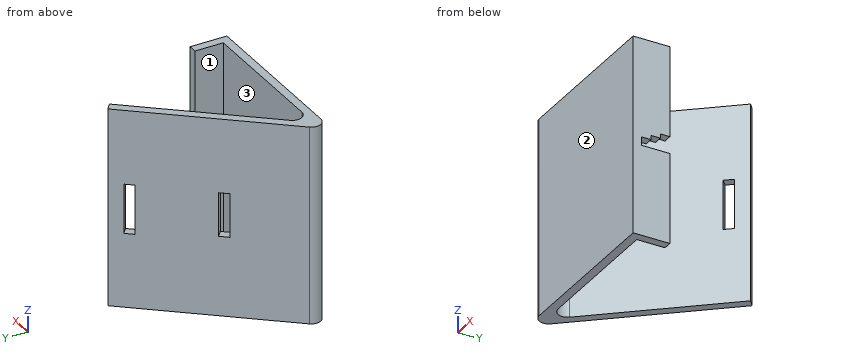
```python
from build123d import *

# Parameters (mm, degrees)
PAD_DEPTH       = 70
SKETCH001_W     = 3.5
SKETCH001_H     = 17.5
SKETCH001_H_2   = 15.5
POCKET_DEPTH    = 34.50505
POCKET001_DEPTH = 5


with BuildPart() as part:
    # Sketch → Pad (new body)
    with BuildSketch(Plane.XY):
        with BuildLine():
            Line((7.250462, 0), (65, 0))
            Line((65, 0), (65, 3))
            Line((65, 3), (65, 13))
            Line((65, 13), (62, 13))
            Line((62, 13), (62, 3))
            Line((62, 3), (13.683983, 3))
            ThreePointArc((11.094028, 8.554176), (10.619805, 4.952097), (13.683983, 3))
            Line((11.094028, 8.554176), (47.293266, 51.694748))
            Line((47.293266, 51.694748), (44.995133, 53.623111))
            Line((4.660507, 5.554176), (44.995133, 53.623111))
            ThreePointArc((4.660507, 5.554176), (4.186285, 1.952097), (7.250462, 0))
        make_face()
    extrude(amount=PAD_DEPTH)

    # Sketch001 (on Face9 of Pad) → Pocket (cut, through all)
    with BuildSketch(Plane(origin=(2.298133, -1.928363, 0), x_dir=(0.642788, 0.766044, 0), z_dir=(0.766044, -0.642788, 0))):
        with Locations((63.25, 35)):
            Rectangle(SKETCH001_W, SKETCH001_H)
        with Locations((33.75, 36)):
            Rectangle(SKETCH001_W, SKETCH001_H_2)
    extrude(amount=-POCKET_DEPTH, mode=Mode.SUBTRACT)

    # Sketch002 (on Face16 of Pocket) → Pocket001 (cut)
    with BuildSketch(Plane.YZ.offset(65)):
        Polygon((3, 35), (3, 32), (13, 32), (13, 38), (9.666667, 38), (9.666667, 36.5), (6.333333, 36.5), (6.333333, 35), align=None)
    extrude(amount=-POCKET001_DEPTH, mode=Mode.SUBTRACT)


solid = part.part
```
Read the model definition and answer for the solid it produces. Units are mm, in the model's axes. Face numbers are marked on the shaded views. Give positions to 0.01 mm unless a question says otherwise; leave off trailing zeros. Order: outer loops, then holes, each group sorted by start corner. A loop starts at its lowest first (then second) coordinate and runs counter-clockwise, first axis right, second up. Notation, with made-up numbers: (-21, -15) -> (18, -15) arc R19 cw to (18, 7) -> close; hole circle Ø10 at (57.25, 73.25). An arc over 180 degrees is marked (long way). One line per item, written item: value. Start each with the question number.
(1) The part is cut by section A-A (z = 40.5). Determine the outline of the cut face in (x, y), and give its area (3 significant figures).
(2) For a pull along Y with two mould halves and no side action, classify the marked faces 1, 2 and 3 as released by +Y, released by -Y, zero draft, split by the parting line, or undercut.
(3) Straight lines are drawn through the part: L1, parallel to Y at x = 51, z = 44; L2, parallel to Y at x = 24, z = 36; L3, parallel to Y at x = 34, z = 11. For each, find the intervals that lie inside material, in ascending order.
(4) Flat-ended cylindrical pins translate along their axes: P1, Ø15.5, axis at x = 27, z = 30, coming from the +Y side; P2, Ø2, axis at y = 33, z = 14.5, coming from the +X side; P3, Ø8, axis at y = 15.5, z = 32.5, coming from the -X side; P4, Ø0.9, axis at x = 63, y = 7.5, coming from the -Z side. Find the tip coordinate at first contact, or state that the pin passes through.
(5) The part is cut by section C-C (y = 7.5). Determine the outline of the cut face in (x, z), and give its area (3 significant figures).
(6) The part is cut by section D-D (z = 25). Determine the outline of the cut face in (x, y).
(7) The part is cut by section B-B (x = 37.5). Determine the outline of the cut face in (y, z).
Taken from the geometry:
1. outline: (4.66, 5.55) arc R3.38 ccw to (7.25, 0) -> (65, 0) -> (65, 13) -> (62, 13) -> (62, 3) -> (13.68, 3) arc R3.38 cw to (11.09, 8.55) -> (22.87, 22.59) -> (20.57, 24.51) -> close; (22.82, 27.19) -> (25.12, 25.27) -> (41.83, 45.18) -> (39.53, 47.11) -> close; (41.78, 49.79) -> (44.08, 47.86) -> (47.29, 51.69) -> (45, 53.62) -> close
1. area: 395 mm^2
2. face 1: zero draft
2. face 2: released by -Y
2. face 3: undercut
3. L1: 0 to 3
3. L2: 0 to 3, 26.2 to 28.6
3. L3: 0 to 3, 35.85 to 40.52
4. P1: y = 41.41
4. P2: x = 32.45
4. P3: x = 9.65
4. P4: z = 0
5. outline: (6.29, 0) -> (10.49, 0) -> (10.49, 70) -> (6.29, 70) -> close; (62, 0) -> (65, 0) -> (65, 32) -> (62, 32) -> close; (62, 36.5) -> (65, 36.5) -> (65, 70) -> (62, 70) -> close
5. area: 491 mm^2
6. outline: (4.66, 5.55) arc R3.38 ccw to (7.25, 0) -> (65, 0) -> (65, 13) -> (62, 13) -> (62, 3) -> (13.68, 3) arc R3.38 cw to (11.09, 8.55) -> (47.29, 51.69) -> (45, 53.62) -> close
7. outline: (0, 0) -> (3, 0) -> (3, 70) -> (0, 70) -> close; (40.02, 0) -> (44.69, 0) -> (44.69, 70) -> (40.02, 70) -> close
